Build history of the part. All positions in model axes, mm. A direction names the side the tool comes from. Round coordinates to 2 decimals unless told otherwise and drop trailing zeros. Loops run counter-clockwise (first coordinate to the right, second up) from the corner with the lowest first, then second, coordinate; pieces in that order, holes last. Notation, with made-up numbers: (-8, 2) - (44, 2) arc R25 ccw to (44, 29) - close; hole circle Ø9 at (-24.75, -33). An arc over 180 degrees is marked (long way). Use a Markdown table: item, result.
Autodesk Inventor part; units mm, degrees
ref_plane "YZ Plane" through (0, 0, 0) normal (1, 0, 0) x (0, 1, 0)
ref_plane "XZ Plane" through (0, 0, 0) normal (0, 1, 0) x (-1, 0, 0)
ref_plane "XY Plane" through (0, 0, 0) normal (0, 0, 1) x (1, 0, 0)
ref_plane "Work Plane1" through (0, 0, 0) normal (0, 0, 1) x (1, 0, 0)
sketch "Sketch1" plane through (0, 0, 0) normal (0, 0, 1) x (1, 0, 0)
  circle A0 centre (25.75, 18) radius 1.7
  circle A1 centre (-4.25, 18) radius 1.7
  circle A2 centre (15.75, 18) radius 1.7
  circle A3 centre (25.75, -18) radius 1.7
  circle A4 centre (15.75, -18) radius 1.7
  circle A5 centre (-4.25, -18) radius 1.7
  line L0 (-12.45, 24.7) -> (32.45, 24.7) construction
  line L1 (-12.45, -24.7) -> (-12.45, 24.7)
  line L2 (-12.45, -24.7) -> (32.45, -24.7)
  line L3 (32.45, 24.7) -> (32.45, -24.7)
  circle A6 centre (-2.25, 0) radius 5.2
  circle A7 centre (5.75, -18) radius 1.7
  circle A8 centre (5.75, 18) radius 1.7
  line L4 (10.75, 24.8) -> (30.75, 24.8)
  line L5 (30.75, 24.8) -> (30.75, 13)
  line L6 (30.75, 13) -> (10.75, 13)
  line L7 (10.75, 13) -> (10.75, 24.8)
  point P0 (0, 0)
  dimension "d0" = 5
  dimension "d1" = 5
  dimension "d2" = 5
  dimension "d3" = 0.1
extrude "Extrusion1" add sketch "Sketch1" along normal blind 5 contours L4 L5 L6 L7
sketch "Sketch2" plane through (30.75, 13, 0) normal (1, 0, 0) x (0, 0, -1)
  line L0 (0, 11.8) -> (-5, 11.8)
  line L1 (-5, 11.8) -> (21, 11.8)
  line L2 (21, 11.8) -> (21, 37.8)
  line L3 (21, 37.8) -> (-5, 37.8)
  line L4 (-5, 37.8) -> (-5, 11.8)
  circle A0 centre (8, 24.8) radius 10.65
  circle A1 centre (8, 24.8) radius 13
  line L5 (6.5, 37.7132) -> (6.5, 35.3438)
  line L6 (9.5, 37.7132) -> (9.5, 35.3438)
  line L7 (8, 37.8) -> (8, 24.8) construction
  line L8 (6.5, 35.3438) -> (3.5, 35.3438)
  line L9 (3.5, 35.3438) -> (3.5, 42.7132)
  line L10 (3.5, 42.7132) -> (6.5, 42.7132)
  line L11 (6.5, 42.7132) -> (6.5, 35.3438)
  line L12 (12.5, 35.3438) -> (12.5, 42.7132)
  line L13 (12.5, 42.7132) -> (9.5, 42.7132)
  line L14 (9.5, 42.7132) -> (9.5, 35.3438)
  line L15 (9.5, 35.3438) -> (12.5, 35.3438)
  point P0 (0, -13)
  point P1 (21, 24.8)
  point P2 (-5, 24.8)
  point P3 (21, 24.8)
  point P4 (12.5, 36.9963)
  point P5 (3.5, 36.9963)
  dimension "d6" = 26
  dimension "d7" = 26
  dimension "d8" = 21.3
  dimension "d9" = 3
  dimension "d10" = 3
  dimension "d11" = 5
extrude "Extrusion2" add sketch "Sketch2" against normal blind 5 contours L0 L4 A1 L1 | A1 L2 L1 | A1 L9 L8 A0 L15 L12 | L9 L3 L11 A1 | A1 L5 L8 L9 | L12 L15 L6 A1 | A1 L14 L3 L12 | L9 L10 L11 L3 | L3 L14 L13 L12
sketch "Sketch3" plane through (30.75, 49.9963, -3.5) normal (0, 0, 1) x (1, 0, 0)
  line L0 (0, 5.7169) -> (0, 0)
  line L1 (0, 5.7169) -> (-5, 5.7169)
  line L2 (-5, 0) -> (-5, 5.7169)
  line L3 (0, 0) -> (-5, 0)
  circle A0 centre (-2.5, 2.8584) radius 1.65
  point P0 (-30.75, -49.9963)
  point P1 (-5, 2.8584)
  point P2 (-2.5, 5.7169)
  dimension "d14" = 3.3
extrude "Extrusion3" cut sketch "Sketch3" against normal through all contours A0
equation "\"d6\" = d7"
properties part number "hopper motor holder"
Q1. Cut at A-A, the plane x = 15.75. List the corners of the cut face in (y, z), plus the area to 3 significant figures.
Results found:
| item | result |
|---|---|
| outline | (13, 0) - (16.3, 0) - (16.3, 5) - (13, 5) - close; (19.7, 0) - (24.8, 0) - (24.8, 5) - (19.7, 5) - close |
| area | 42.0 mm2 |
Q2. Pull direction Y, two halves, no side cores. Call faces 1 (the face through (30, 52, -12.5)), 2 (the face through (21, 13, 2)), 3 (the face through (27.034, 53.97, -4.979)): pulls with the +Y half, pulls with the -Y half, needs draft (parallel to the pull), parting line crosses it, or undercut.
Results found:
| item | result |
|---|---|
| face 1 | needs draft |
| face 2 | pulls with the -Y half |
| face 3 | undercut |
Q3. Cut at B-B, the plane y = 18. List the corners of the cut face in (x, z), plus the area to 3 significant figures.
Results found:
| item | result |
|---|---|
| outline | (10.75, 0) - (14.05, 0) - (14.05, 5) - (10.75, 5) - close; (17.45, 0) - (24.05, 0) - (24.05, 5) - (17.45, 5) - close; (27.45, 0) - (30.75, 0) - (30.75, 5) - (27.45, 5) - close |
| area | 66.0 mm2 |
Q4. Which spindle directions (+Z, -Z, +X, -X, +Y, -Y) get a long thin tool onto all of the face, cutting with end or side? Do faces 4 (the face through (25.75, 27.7, -4.1)), 5 (the face through (28, 24.8, -11)), 6 (the face through (29, 51, -6.5)), 7 (the face through (30, 52, -3.5)). Say none if no direction does.
Results found:
| item | result |
|---|---|
| face 4 | +Z, -Z, -X, +Y |
| face 5 | -Z, +X, -X, -Y |
| face 6 | +X, -X, +Y |
| face 7 | +Z, +X, -X, +Y |
Q5. Drop flat-ended pins along their axis: pin 1 (5.5 mm diameter, centred on x = 28, y = 51.5, fed in from +Z); pin 2 (5.5 mm diameter, centred on x = 28.25, y = 52.85, fed in from +Z); pin 3 (5.5 mm diameter, centred on x = 15.75, y = 18, fed in from -Z); pin 4 (1.5 mm diameter, centred on y = 24, z = -11.5, fed in from +X). Give the stop position or say it passes through.
Results found:
| item | result |
|---|---|
| pin 1 | stops at z = -0.99 |
| pin 2 | stops at z = -3.5 |
| pin 3 | stops at z = 0 |
| pin 4 | passes through |
Q6. Cut at C-C, the plane z = 0.75. List the corners of the cut face in (x, y).
Results found:
| item | result |
|---|---|
| outline | (10.75, 13) - (30.75, 13) - (30.75, 31.73) - (25.75, 31.73) - (25.75, 24.8) - (10.75, 24.8) - close; (25.75, 43.87) - (30.75, 43.87) - (30.75, 47.41) - (25.75, 47.41) - close; hole circle Ø3.4 at (15.75, 18); hole circle Ø3.4 at (25.75, 18) |
Q7. Cut at D-D, the plane y = 49. List the corners of the cut face in (x, z), plus the area to 3 significant figures.
Results found:
| item | result |
|---|---|
| outline | (25.75, -14.6) - (30.75, -14.6) - (30.75, -9.5) - (25.75, -9.5) - close; (25.75, -6.5) - (30.75, -6.5) - (30.75, -1.4) - (25.75, -1.4) - close |
| area | 51.0 mm2 |
Q8. Probe line 1 (Y direction, x = 28.25, z = -10.5); line 2 (Y direction, x = 15.75, z = 2.45); line 3 (Z direction, x = 16.75, y = 24.5). List the from-to ranges inside material, lowest first.
Results found:
| item | result |
|---|---|
| line 1 | y = 24.8 to 27.45, 48.15 to 51.2, 54.5 to 55.71 |
| line 2 | y = 13 to 16.3, 19.7 to 24.8 |
| line 3 | z = 0 to 5 |
